Read the model definition and answer for the solid it produces. Units are mm, in the model's axes. A direction names the side the tool comes from. Round coordinates to 2 decimals unless told otherwise and drop trailing zeros. Order: outer loops, then holes, each group sorted by start corner. A loop starts at its lowest first (then second) coordinate and runs counter-clockwise, first axis right, second up. Notation, with made-up numbers: (-29.5, 18.25) - (-2.5, 18.25) arc R23 cw to (-2.5, 41.25) - close; hole circle Ø4 at (32, 41). An arc over 180 degrees is marked (long way). Put each result on its own line as item: value. Start each with the question number.
Q1. Find the intervals of material crossed by line 1 along X through (y, z) = (3, 19); line 2 along Z through (x, y) = (-1, 3); line 3 along X through (y, z) = (5.25, 24), in increasing order. Write a range as from..to.
Q2. Section C-C on x = -29.5 is taken. Give the vertices of the cut face in (y, z), then the cut area to 3 significant figures.
Q3. Which of the six approach directions +Z, -Z, +X, -X, +Y, -Y give full straight-line access (tool end or side, diameter ignored) to faces 1 (the face through (58, 3, -34.5)), 2 (the face through (-0.521, 3.131, 48.306))?
Q4. Section B-B on x = -54.5 is taken. Give the vertices of the cut face in (y, z), then the cut area to 3 significant figures.
Q5. Section D-D on y = 3.75 is taken. State how many separate pieces and enclosed holes the cut face has, then the cut area to 3 significant figures.
Q6. Section A-A on z = 0 is taken. Give the vertices of the cut face in (x, y), then the cut area to 3 significant figures.
Q7. Each of these flat-tipped pins is pushed along its axis until it touches: pin 1 Ø1.8 at (x, z) = (9.16, -11.1) entering from +Y; pin 2 Ø2 at (y, z) = (2.5, -15.5) entering from -X (3 decimals); pin 3 Ø1.5 at (x, y) = (-54, 3) entering from +Z. Where does it stop, or does it pass through?
from build123d import *

# Parameters (mm, degrees)
SKETCH1_R           = 1.5
BOSS_EXTRUDE2_DEPTH = 6.35


with BuildPart() as part:
    # Sketch1 → Boss-Extrude2 (new body)
    with BuildSketch(Plane(origin=(0, 0, 0), x_dir=(1, 0, 0), z_dir=(0, 1, 0))):
        with BuildLine():
            ThreePointArc((35.49727084, -66.067721036), (0, 75), (-35.49727084, -66.067721036))
            ThreePointArc((-35.49727084, -66.067721036), (-33.357679643, -66.33740492), (-31.589980006, -65.102164912))
            ThreePointArc((-31.589980006, -65.102164912), (0, -48.302004425), (31.589980006, -65.102164912))
            ThreePointArc((31.589980006, -65.102164912), (33.357679643, -66.33740492), (35.49727084, -66.067721036))
        make_face()
        with Locations((-13.608916499, -21.183093811)):
            Circle(SKETCH1_R, mode=Mode.SUBTRACT)
        with Locations((-46.011477091, 28.075890486)):
            Circle(SKETCH1_R, mode=Mode.SUBTRACT)
        with Locations((13.608916499, -21.183093811)):
            Circle(SKETCH1_R, mode=Mode.SUBTRACT)
        with Locations((23.852486199, -41.694616163)):
            Circle(SKETCH1_R, mode=Mode.SUBTRACT)
        with Locations((-40.910067426, 11.1)):
            Circle(SKETCH1_R, mode=Mode.SUBTRACT)
        with Locations((-40.910067426, -11.1)):
            Circle(SKETCH1_R, mode=Mode.SUBTRACT)
        with Locations((-9.160067426, -11.1)):
            Circle(SKETCH1_R, mode=Mode.SUBTRACT)
        with Locations((-9.160067426, 11.1)):
            Circle(SKETCH1_R, mode=Mode.SUBTRACT)
        with Locations((9.160067426, 11.1)):
            Circle(SKETCH1_R, mode=Mode.SUBTRACT)
        with Locations((9.160067426, -11.1)):
            Circle(SKETCH1_R, mode=Mode.SUBTRACT)
        with Locations((40.910067426, -11.1)):
            Circle(SKETCH1_R, mode=Mode.SUBTRACT)
        with Locations((40.910067426, 11.1)):
            Circle(SKETCH1_R, mode=Mode.SUBTRACT)
        with Locations((-23.852486199, -41.694616163)):
            Circle(SKETCH1_R, mode=Mode.SUBTRACT)
        with Locations((19.397913834, 18.186588214)):
            Circle(SKETCH1_R, mode=Mode.SUBTRACT)
        with Locations((-40.277379234, -25.14022965)):
            Circle(SKETCH1_R, mode=Mode.SUBTRACT)
        with Locations((40.277379234, -25.14022965)):
            Circle(SKETCH1_R, mode=Mode.SUBTRACT)
        with Locations((26.163250867, 37.1696126)):
            Circle(SKETCH1_R, mode=Mode.SUBTRACT)
        with Locations((46.011477091, 28.075890486)):
            Circle(SKETCH1_R, mode=Mode.SUBTRACT)
        with Locations((10.027203595, 39.91869143)):
            Circle(SKETCH1_R, mode=Mode.SUBTRACT)
        with Locations((0, -39.659190322)):
            Circle(SKETCH1_R, mode=Mode.SUBTRACT)
        with Locations((-10.027203595, 39.91869143)):
            Circle(SKETCH1_R, mode=Mode.SUBTRACT)
        with Locations((-33.059737365, -55.383244446)):
            Circle(SKETCH1_R, mode=Mode.SUBTRACT)
        with Locations((-33.059737365, 55.383244446)):
            Circle(SKETCH1_R, mode=Mode.SUBTRACT)
        with Locations((33.059737365, -55.383244446)):
            Circle(SKETCH1_R, mode=Mode.SUBTRACT)
        with Locations((0, 15.543589551)):
            Circle(SKETCH1_R, mode=Mode.SUBTRACT)
        with Locations((-26.163250867, 37.1696126)):
            Circle(SKETCH1_R, mode=Mode.SUBTRACT)
        with Locations((-19.397913834, 18.186588214)):
            Circle(SKETCH1_R, mode=Mode.SUBTRACT)
        with Locations((33.059737365, 55.383244446)):
            Circle(SKETCH1_R, mode=Mode.SUBTRACT)
        with BuildLine():
            Line((51.410067426, -34), (51.410067426, 34))
            ThreePointArc((51.410067426, 34), (51.556514035, 34.353553391), (51.910067426, 34.5))
            Line((51.910067426, 34.5), (63.910067426, 34.5))
            ThreePointArc((63.910067426, 34.5), (64.263620817, 34.353553391), (64.410067426, 34))
            Line((64.410067426, 34), (64.410067426, -34))
            ThreePointArc((64.410067426, -34), (64.263620817, -34.353553391), (63.910067426, -34.5))
            Line((63.910067426, -34.5), (51.910067426, -34.5))
            ThreePointArc((51.910067426, -34.5), (51.556514035, -34.353553391), (51.410067426, -34))
        make_face(mode=Mode.SUBTRACT)
        with BuildLine():
            Line((-63.910067426, -34.5), (-51.910067426, -34.5))
            ThreePointArc((-51.910067426, -34.5), (-51.556514035, -34.353553391), (-51.410067426, -34))
            Line((-51.410067426, -34), (-51.410067426, 34))
            ThreePointArc((-51.410067426, 34), (-51.556514035, 34.353553391), (-51.910067426, 34.5))
            Line((-51.910067426, 34.5), (-63.910067426, 34.5))
            ThreePointArc((-63.910067426, 34.5), (-64.263620817, 34.353553391), (-64.410067426, 34))
            Line((-64.410067426, 34), (-64.410067426, -34))
            ThreePointArc((-64.410067426, -34), (-64.263620817, -34.353553391), (-63.910067426, -34.5))
        make_face(mode=Mode.SUBTRACT)
        with BuildLine():
            ThreePointArc((-5.853899988, 64.744946271), (0.003726822, 68.153564176), (5.857575472, 64.738461857))
            ThreePointArc((5.857575472, 64.738461857), (10.16, 61.422565207), (5.857575472, 58.106668557))
            ThreePointArc((5.857575472, 58.106668557), (0.003726822, 54.691566239), (-5.853899988, 58.100184144))
            ThreePointArc((-5.853899988, 58.100184144), (-10.167207264, 61.422565207), (-5.853899988, 64.744946271))
        make_face(mode=Mode.SUBTRACT)
    extrude(amount=BOSS_EXTRUDE2_DEPTH)


solid = part.part
Findings:
1. line 1: -72.55..-64.41, -51.41..51.41, 64.41..72.55
1. line 2: -74.99..-68.08, -54.77..-16.66, -14.43..38.54, 40.78..48.32
1. line 3: -71.06..-64.41, -51.41..-41.25, -39.3..39.3, 41.25..51.41, 64.41..71.06
2. outline: (0, -68.95) - (6.35, -68.95) - (6.35, 62.29) - (0, 62.29) - close
2. area: 833 mm2
3. face 1: +Y, -Y
3. face 2: +Z, +Y, -Y
4. outline: (0, -51.52) - (6.35, -51.52) - (6.35, -34.5) - (0, -34.5) - close; (0, 34.5) - (6.35, 34.5) - (6.35, 51.52) - (0, 51.52) - close
4. area: 216 mm2
5. separate pieces: 1
5. enclosed holes: 31
5. area: 14,300 mm2
6. outline: (-75, 0) - (-64.41, 0) - (-64.41, 6.35) - (-75, 6.35) - close; (-51.41, 0) - (51.41, 0) - (51.41, 6.35) - (-51.41, 6.35) - close; (64.41, 0) - (75, 0) - (75, 6.35) - (64.41, 6.35) - close
6. area: 787 mm2
7. pin 1: through
7. pin 2: x = -73.585
7. pin 3: z = 52.82
